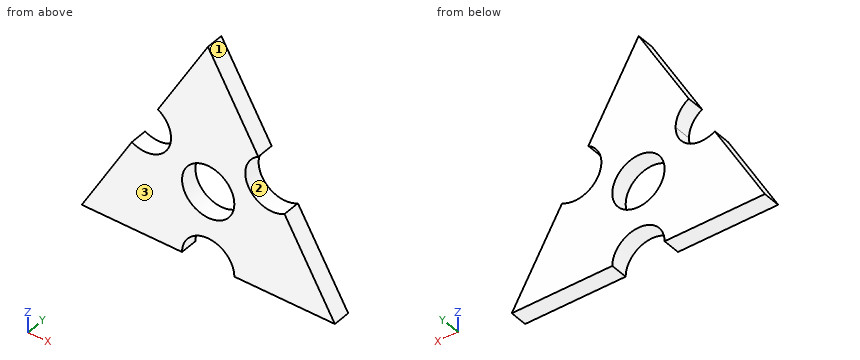
from build123d import *

# Parameters (mm, degrees)
F0_R     = 7.62
F1_DEPTH = 5.08


with BuildPart() as f1:
    # F0 (on Front) → F1 (new body)
    with BuildSketch(Plane.XZ):
        with BuildLine():
            Line((7.61999, -21.275166), (36.905502, -21.227668))
            Line((36.905502, -21.227668), (22.238923, 4.080709))
            ThreePointArc((22.238923, 4.080709), (11.8253, 6.852936), (14.597528, 17.26656))
            Line((14.597528, 17.26656), (-0.069051, 42.574937))
            Line((-0.069051, 42.574937), (-14.653459, 17.219118))
            ThreePointArc((-14.653459, 17.219118), (-11.856729, 14.429184), (-10.832751, 10.613834))
            ThreePointArc((-10.832751, 10.613834), (-14.637401, 4.017812), (-22.252043, 4.00855))
            Line((-22.252043, 4.00855), (-36.836451, -21.347268))
            Line((-36.836451, -21.347268), (-7.61999, -21.299883))
            ThreePointArc((-7.61999, -21.299883), (-0.012359, -13.667534), (7.61999, -21.275166))
        make_face()
        Circle(F0_R, mode=Mode.SUBTRACT)
    extrude(amount=F1_DEPTH)


solid = f1.part
Read the model definition and answer for the solid it produces. Units are mm, in the model's axes. Face numbers are marked on the shaded views. Round coordinates to 2 decimals unless told otherwise and drop trailing zeros. Loops run counter-clockwise (first coordinate to the right, second up) from the corner with the lowest first, then second, coordinate; pieces in that order, holes last. Notation, with made-up numbers: (68, 9.5) - (73, 9.5) arc R18 ccw to (73, 34.5) - close; hole circle Ø4 at (-25.75, 67.5). An arc over 180 degrees is marked (long way). One line per question, with ' | ' between items. Start each with the question number.
Q1. For a pull along Z with two mould halves and no side action, classify the marked faces 1, 2 and 3 as +Z half, -Z half, draft (parallel to the pull), parting line (faces both ways), or undercut.
Q2. Section D-D on x = -30.5 is taken. Give the vertices of the cut face in (y, z).
Q3. Section A-A on y = -4.05 is taken. Give the vertices of the cut face in (x, z).
Q4. Find the intervals of material crossed by L1, parallel to Z at x = 0, y = -1.7; L2, parallel to X at y = -1.8, z = 6; L3, parallel to Z at x = 27.5, y = -2.8, in increasing order.
Q5. A flat-ended cylindrical pin translates along its axis: pin 1 (9 mm diameter, centred on x = 0, z = 0, fed in from +Y). Find the tip coordinate at first contact, or state that the pin passes through.
Q6. Section B-B on z = -6 is taken. Give the vertices of the cut face in (x, y), plus the area to 3 significant figures.
Q7. Section C-C on z = -16 is taken. Give the vertices of the cut face in (x, y).
Established:
1) face 1: +Z half | face 2: undercut | face 3: draft
2) outline: (-5.08, -21.34) - (0, -21.34) - (0, -10.33) - (-5.08, -10.33) - close
3) outline: (-36.84, -21.35) - (-7.62, -21.3) arc R7.62 cw to (7.62, -21.28) - (36.91, -21.23) - (22.24, 4.08) arc R7.62 cw to (14.6, 17.27) - (-0.07, 42.57) - (-14.65, 17.22) arc R7.62 cw to (-10.83, 10.61) arc R7.62 cw to (-22.25, 4.01) - close; hole circle Ø15.24 at (0, 0)
4) L1: -13.67 to -7.62, 7.62 to 42.46 | L2: -12.39 to -4.7, 4.7 to 12.4 | L3: -21.24 to -5
5) pin 1: through
6) outline: (-28.01, -5.08) - (-4.7, -5.08) - (-4.7, 0) - (-28.01, 0) - close; (4.7, -5.08) - (28.08, -5.08) - (28.08, 0) - (4.7, 0) - close | area: 237 mm²
7) outline: (-33.76, -5.08) - (-5.49, -5.08) - (-5.49, 0) - (-33.76, 0) - close; (5.49, -5.08) - (33.88, -5.08) - (33.88, 0) - (5.49, 0) - close
